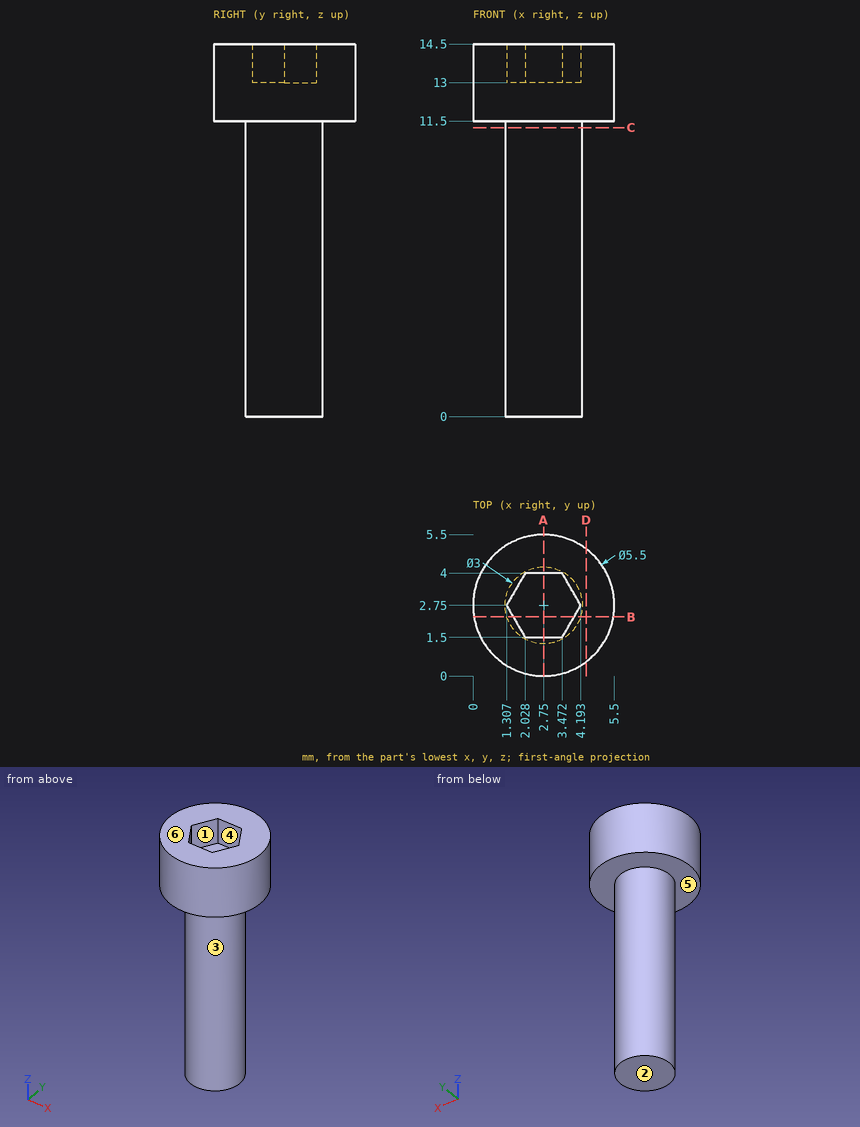
Print and shaded views of the part. All mm, measured from the part's lowest x, y and z. A direction names the side the tool comes from. Give positions to 0.01 mm unless a question says otherwise; leave off trailing zeros. Write each loop counter-clockwise with the first axis right and the second up, starting at its lowest first coordinate (ties: lowest second). Pieces come first, ordered by that corner, then holes. Notation, with made-up numbers: (-23.5, 51.25) -> (-16.5, 51.25) arc R27 cw to (-16.5, 88.25) -> close; hole circle Ø3 at (-11.75, 32). An arc over 180 degrees is marked (long way). Write each question's results on one line, items separated by ' | '.
1. Two-plate mould, pull along X, no slides. Class the marked faces 1, 2, 3 and 4: pulls with the +X half, pulls with the -X half, needs draft (parallel to the pull), parting line crosses it, or undercut.
Geometry check:
face 1: undercut | face 2: needs draft | face 3: parting line crosses it | face 4: undercut
2. Cut at A-A, the plane x = 2.75. Write the cut outline in (y, z).
Geometry check:
outline: (0, 11.5) -> (1.25, 11.5) -> (1.25, 0) -> (4.25, 0) -> (4.25, 11.5) -> (5.5, 11.5) -> (5.5, 14.5) -> (4, 14.5) -> (4, 13) -> (1.5, 13) -> (1.5, 14.5) -> (0, 14.5) -> close
3. Cut at D-D, the plane x = 4.4. Write the cut outline in (y, z).
Geometry check:
outline: (0.55, 11.5) -> (4.95, 11.5) -> (4.95, 14.5) -> (0.55, 14.5) -> close
4. Which spindle directions (+Z, -Z, +X, -X, +Y, -Y) get a long thin tool onto all of the face, cutting with end or side? Do the marked faces 5 and 6. Say none if no direction does.
Geometry check:
face 5: -Z | face 6: +Z, +X, -X, +Y, -Y
5. Cut at C-C, the plane z = 11.25. Write the cut outline in (x, y).
Geometry check:
outline: circle Ø3 at (2.75, 2.75)
6. Cut at B-B, the plane y = 2.3. Write the cut outline in (x, z).
Geometry check:
outline: (0.04, 11.5) -> (1.32, 11.5) -> (1.32, 0) -> (4.18, 0) -> (4.18, 11.5) -> (5.46, 11.5) -> (5.46, 14.5) -> (3.93, 14.5) -> (3.93, 13) -> (1.57, 13) -> (1.57, 14.5) -> (0.04, 14.5) -> close
7. Wall check: probe 1 along Y at (x, z) = (3.15, 7.5) (1 decimal); probe 2 along Z at (x, y) = (5.35, 3.3); probe 3 along Z at (x, y) = (2.9, 2.1). Give the ranges that are in metal, low to high. Write a range as [from, to].
Geometry check:
probe 1: [1.3, 4.2] | probe 2: [11.5, 14.5] | probe 3: [0, 13]
